from build123d import *

# Parameters (mm, degrees)
F0_W       = 50
F0_H       = 10
F1_DEPTH   = 12.5
F2_W       = 6
F2_H       = 12.5
F3_DEPTH   = 5
F4_W       = 2
F4_H       = 7
F5_W       = 2
F5_H       = 7
F8_D       = 2.4
F8_ON_F5_D = 2.4


with BuildPart() as f1:
    # F0 (on Front) → F1 (new body)
    with BuildSketch(Plane.XZ):
        Rectangle(F0_W, F0_H)
    extrude(amount=F1_DEPTH)

    # F2 (on face) → F3 (cut)
    with BuildSketch(Plane.XY.offset(5)):
        with Locations((-15, -6.25)):
            Rectangle(F2_W, F2_H)
        with Locations((15, -6.25)):
            Rectangle(F2_W, F2_H)
    extrude(amount=-F3_DEPTH, mode=Mode.SUBTRACT)

    # F4 (on face) → F6 (revolve, cut)
    with BuildSketch(Plane.XY):
        with Locations((-14, -3.5)):
            Rectangle(F4_W, F4_H)
    revolve(axis=Axis((-15, -7.6616932638, 0), (0, -1, 0)), mode=Mode.SUBTRACT)

    # F5 (on face) → F7 (revolve, cut)
    with BuildSketch(Plane.XY):
        with Locations((16, -3.5)):
            Rectangle(F5_W, F5_H)
    revolve(axis=Axis((15, -9.4139035791, 0), (0, -1, 0)), mode=Mode.SUBTRACT)

    # F8 (through all)
    with Locations(Plane.XY):
        with Locations((-15, -9)):
            Hole(F8_D / 2)

    # F8 on F5 (through all)
    with Locations(Plane.XY):
        with Locations((15, -9)):
            Hole(F8_ON_F5_D / 2)


solid = f1.part
For this review, take the finished solid that the model builds, in its own axes (mm). A direction names the side the tool comes from. Round coordinates to 2 decimals unless told otherwise and drop trailing zeros. Loops run counter-clockwise (first coordinate to the right, second up) from the corner with the lowest first, then second, coordinate; pieces in that order, holes last. Notation, with made-up numbers: (60.25, -4.75) - (69.25, -4.75) arc R18 ccw to (69.25, 9.25) - close; hole circle Ø11 at (7.5, 52). An arc over 180 degrees is marked (long way). Put each result on its own line as item: value. Start each with the question number.
1. Insertion check: P1, Ø1.9, axis at x = 15, y = -9, coming from the +Z side; P2, Ø0.6, axis at x = -15, z = -1, coming from the +Y side. Each pin has a flat end and moves straight along its axis. Give the tip position at first contact, or say it passes through.
2. Consider section A-A on x = -15. State the section outline as (y, z) points.
3. Mouldability with a two-part tool opening along X and no side actions: class faces 4 (the flat face through (-15, -7.6, 0)), 5 (the cylindrical face through (-16.11, -9.46, -2.53)), 6 (the flat face through (25, -6, 0)), 7 (the flat face through (0, 0, 0)) as +X half, -X half, draft (parallel to the pull), parting line (faces both ways), or undercut.
4. For probe 1 along Y at (x, z) = (15, -3.7); probe 2 along X at (y, z) = (-9.75, 4); probe 3 along X at (y, z) = (-1.5, -1.75), list the stretches that pass through material, from the lowest coordinate up. Write a range as [from, to].
5. For faces 1 (the cylindrical face through (15, -3, -2)), 2 (the flat face through (-25, -6, 0)), 3 (the flat face through (-18, -6, 3)), list the 3-axis set-ups (+Z, -Z, +X, -X, +Y, -Y) from which the entire face can be reached by the end or side of a thin tool; tool diameter is ignored.
6. Consider section C-C on y = -9. State the section outline as (x, z) points, plus the area to 3 significant figures.
7. Consider section B-B on z = 0.5. State the section outline as (x, y) points, plus the area to 3 significant figures.
8. Consider section D-D on y = -3.5. State the section outline as (x, z) points, plus the area to 3 significant figures.
Result sheet:
1. P1: through
1. P2: y = -7
2. outline: (-12.5, -5) - (-10.2, -5) - (-10.2, 0) - (-12.5, 0) - close; (-7.8, -5) - (0, -5) - (0, -2) - (-7, -2) - (-7, 0) - (-7.8, 0) - close
3. face 4: undercut
3. face 5: undercut
3. face 6: +X half
3. face 7: draft
4. probe 1: [-12.5, -10.2], [-7.8, 0]
4. probe 2: [-25, -18], [-12, 12], [18, 25]
4. probe 3: [-25, -15.97], [-14.03, 14.03], [15.97, 25]
5. face 1: +Z, +Y
5. face 2: +Z, -Z, -X, +Y, -Y
5. face 3: +Z, +Y, -Y
6. outline: (-25, -5) - (-16.2, -5) - (-16.2, 0) - (-18, 0) - (-18, 5) - (-25, 5) - close; (-13.8, -5) - (13.8, -5) - (13.8, 0) - (12, 0) - (12, 5) - (-12, 5) - (-12, 0) - (-13.8, 0) - close; (16.2, -5) - (25, -5) - (25, 5) - (18, 5) - (18, 0) - (16.2, 0) - close
6. area: 416 mm^2
7. outline: (-25, -12.5) - (-18, -12.5) - (-18, 0) - (-25, 0) - close; (-12, -12.5) - (12, -12.5) - (12, 0) - (-12, 0) - close; (18, -12.5) - (25, -12.5) - (25, 0) - (18, 0) - close
7. area: 475 mm^2
8. outline: (-25, -5) - (25, -5) - (25, 5) - (18, 5) - (18, 0) - (17, 0) arc R2 cw to (13, 0) - (12, 0) - (12, 5) - (-12, 5) - (-12, 0) - (-13, 0) arc R2 cw to (-17, 0) - (-18, 0) - (-18, 5) - (-25, 5) - close
8. area: 427 mm^2
